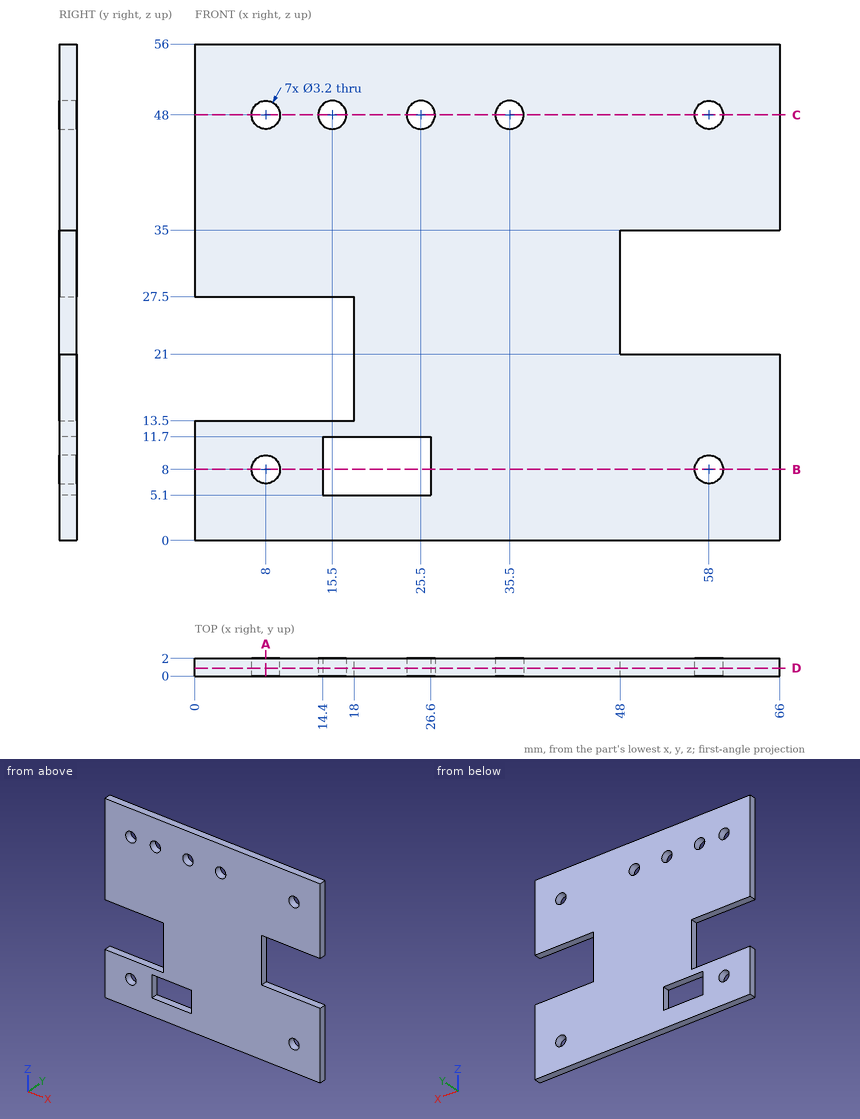
Design review of the part shown in the three views and the two pictorial views. Dimensions are in mm from the part's minimum x, y and z. Round coordinates to 2 decimals unless told otherwise and drop trailing zeros. Write each loop counter-clockwise with the first axis right and the second up, starting at its lowest first coordinate (ties: lowest second). Pieces come first, ordered by that corner, then holes. Notation, with made-up numbers: (57, 60) -> (98, 60) arc R17 ccw to (98, 72) -> close; hole circle Ø1 at (63, 47.25). An arc over 180 degrees is marked (long way). Answer as a JSON object with one key per item and string values.
1. We need section D-D on y = 0.9. State how many separate pieces and enclosed holes the cut face has, and give its area (4 significant figures).
Results found:
{"separate pieces": "1", "enclosed holes": "8", "area": "3,055 mm^2"}
2. We need section A-A on x = 8. State the section outline as (y, z) points, and give its area (3 significant figures).
Results found:
{"outline": "(0, 0) -> (2, 0) -> (2, 6.4) -> (0, 6.4) -> close; (0, 9.6) -> (2, 9.6) -> (2, 13.5) -> (0, 13.5) -> close; (0, 27.5) -> (2, 27.5) -> (2, 46.4) -> (0, 46.4) -> close; (0, 49.6) -> (2, 49.6) -> (2, 56) -> (0, 56) -> close", "area": "71.2 mm^2"}
3. We need section C-C on z = 48. State the section outline as (x, y) points.
Results found:
{"outline": "(0, 0) -> (6.4, 0) -> (6.4, 2) -> (0, 2) -> close; (9.6, 0) -> (13.9, 0) -> (13.9, 2) -> (9.6, 2) -> close; (17.1, 0) -> (23.9, 0) -> (23.9, 2) -> (17.1, 2) -> close; (27.1, 0) -> (33.9, 0) -> (33.9, 2) -> (27.1, 2) -> close; (37.1, 0) -> (56.4, 0) -> (56.4, 2) -> (37.1, 2) -> close; (59.6, 0) -> (66, 0) -> (66, 2) -> (59.6, 2) -> close"}
4. To check wall thickness, follow line 1 along X through (y, z) = (1.25, 8); line 2 along X through (y, z) = (1.3, 48); line 3 along Z through (x, y) = (54.5, 1.9). State the ranges of each line that lie inside material, in increasing order.
Results found:
{"line 1": "x = 0 to 6.4, 9.6 to 14.4, 26.6 to 56.4, 59.6 to 66", "line 2": "x = 0 to 6.4, 9.6 to 13.9, 17.1 to 23.9, 27.1 to 33.9, 37.1 to 56.4, 59.6 to 66", "line 3": "z = 0 to 21, 35 to 56"}
5. Clearance check with flat-ended pins moving along their axes: pin 1 (1.9 mm diameter, centred on x = 35.5, z = 48, fed in from +Y); pin 2 (0.6 mm diameter, centred on y = 1, z = 31, fed in from +X). State where each tip first meets the part, or that it passes through.
Results found:
{"pin 1": "passes through", "pin 2": "stops at x = 48"}
6. We need section B-B on z = 8. State the section outline as (x, y) points.
Results found:
{"outline": "(0, 0) -> (6.4, 0) -> (6.4, 2) -> (0, 2) -> close; (9.6, 0) -> (14.4, 0) -> (14.4, 2) -> (9.6, 2) -> close; (26.6, 0) -> (56.4, 0) -> (56.4, 2) -> (26.6, 2) -> close; (59.6, 0) -> (66, 0) -> (66, 2) -> (59.6, 2) -> close"}
